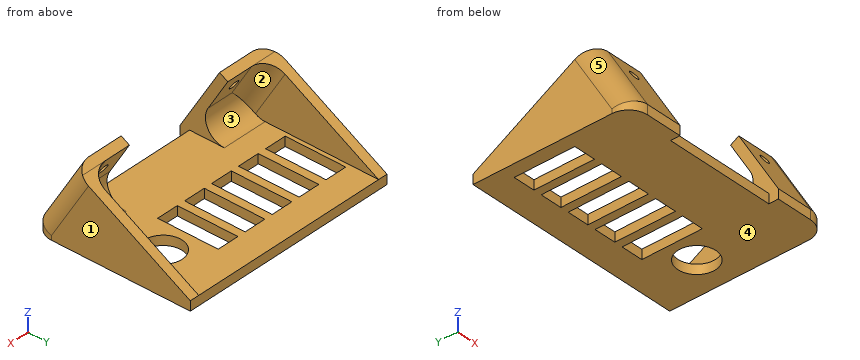
```python
from build123d import *

# Parameters (mm, degrees)
F3_W      = 7
F3_H      = 19.2
F3_R      = 6
F4_DEPTH  = 3
F7_DEPTH  = 3
F8_START  = -67
F8_DEPTH  = 3
F9_START  = -52.5
F9_DEPTH  = 17.5
F10_DEPTH = 17.5
F11_R     = 6
F13_R     = 1.5
F14_DEPTH = 5


with BuildPart() as f4:
    # F3 (on Top) → F4 (new body)
    with BuildSketch(Plane.XY):
        Polygon((35, 25), (-35, 25), (-35, -25), (-17.5, -25), (-17.5, -22), (17.5, -22), (17.5, -25), (35, -25), align=None)
        with Locations((-27.2, 6.1666666667)):
            Rectangle(F3_W, F3_H, mode=Mode.SUBTRACT)
        with Locations((-17.6, 6.1666666667)):
            Rectangle(F3_W, F3_H, mode=Mode.SUBTRACT)
        with Locations((-8, 6.1666666667)):
            Rectangle(F3_W, F3_H, mode=Mode.SUBTRACT)
        with Locations((1.6, 6.1666666667)):
            Rectangle(F3_W, F3_H, mode=Mode.SUBTRACT)
        with Locations((11.2, 6.1666666667)):
            Rectangle(F3_W, F3_H, mode=Mode.SUBTRACT)
        with Locations((23.5, 6.1666666667)):
            Circle(F3_R, mode=Mode.SUBTRACT)
    extrude(amount=F4_DEPTH)

    # F6 (on offset) → F7 (join)
    with BuildSketch(Plane.YZ.offset(35)):
        Polygon((-12.4875, 24.0638871947), (-25, 3), (-21.5106155706, 3), (-9.871334024, 22.5938871947), align=None)
        Polygon((-9.871334024, 22.5938871947), (-21.5106155706, 3), (25, 3), align=None)
    extrude(amount=-F7_DEPTH)

    # F6 (on offset) → F8 (join)
    with BuildSketch(Plane.YZ.offset(35).offset(F8_START)):
        Polygon((-12.4875, 24.0638871947), (-25, 3), (-21.5106155706, 3), (-9.871334024, 22.5938871947), align=None)
        Polygon((-9.871334024, 22.5938871947), (-21.5106155706, 3), (25, 3), align=None)
    extrude(amount=-F8_DEPTH)

    # F6 (on offset) → F9 (join)
    with BuildSketch(Plane.YZ.offset(35).offset(F9_START)):
        Polygon((-12.4875, 24.0638871947), (-25, 3), (-21.5106155706, 3), (-9.871334024, 22.5938871947), align=None)
    extrude(amount=-F9_DEPTH)

    # F6 (on offset) → F10 (join)
    with BuildSketch(Plane.YZ.offset(35)):
        Polygon((-12.4875, 24.0638871947), (-25, 3), (-21.5106155706, 3), (-9.871334024, 22.5938871947), align=None)
    extrude(amount=-F10_DEPTH)

    # F11
    f11_edges = [f4.edges().sort_by_distance(p)[0] for p in [
        (32, -15.690975, 12.796944),
        (-32, -15.690975, 12.796944),
        (-24.75, -21.510616, 3),
        (24.75, -21.510616, 3),
        (35, -18.74375, 13.531944),
        (-35, -18.74375, 13.531944),
        (-35, -25, 1.5),
        (35, -25, 1.5),
    ]]
    fillet(f11_edges, radius=F11_R)

    # F13 (on offset) → F14 (cut)
    with BuildSketch(Plane(origin=(0, -19.7965335432, 11.7596587786), x_dir=(1, 0, 0), z_dir=(0, -0.8597504977, 0.5107142857))):
        with Locations((-23.25, 8.1863943504)):
            Circle(F13_R)
        with Locations((23.25, 8.1863943504)):
            Circle(F13_R)
    extrude(amount=-F14_DEPTH, mode=Mode.SUBTRACT)


solid = f4.part
```
Could you check a few things on this model? Use its own coordinates, in mm. Face numbers are marked on the shaded views. A direction names the side the tool comes from. Round coordinates to 2 decimals unless told otherwise and drop trailing zeros. Loops run counter-clockwise (first coordinate to the right, second up) from the corner with the lowest first, then second, coordinate; pieces in that order, holes last. Notation, with made-up numbers: (-16, 15.25) -> (35, 15.25) arc R19 cw to (35, 35.25) -> close; hole circle Ø11 at (25, -30.75). An arc over 180 degrees is marked (long way). One line per question, with ' | ' between items.
(1) For the marked faces 1 and 2, which set-ups out of +Z, -Z, +X, -X, +Y, -Y let a thin tool reach every point of the face, with its end or its side?
Model answer:
face 1: +Z, -Z, +X, +Y, -Y | face 2: +Y
(2) If we section it at C-C on y = 13: List the corners of the cut face in (x, z) for me.
Model answer:
outline: (-35, 0) -> (-30.7, 0) -> (-30.7, 3) -> (-32, 3) -> (-32, 9.74) -> (-35, 9.74) -> close; (-23.7, 0) -> (-21.1, 0) -> (-21.1, 3) -> (-23.7, 3) -> close; (-14.1, 0) -> (-11.5, 0) -> (-11.5, 3) -> (-14.1, 3) -> close; (-4.5, 0) -> (-1.9, 0) -> (-1.9, 3) -> (-4.5, 3) -> close; (5.1, 0) -> (7.7, 0) -> (7.7, 3) -> (5.1, 3) -> close; (14.7, 0) -> (35, 0) -> (35, 9.74) -> (32, 9.74) -> (32, 3) -> (14.7, 3) -> close
(3) If we section it at A-A on x = -20: List the corners of the cut face in (y, z) for me, and give its area (3 significant figures).
Model answer:
outline: (-25, 0) -> (-3.43, 0) -> (-3.43, 3) -> (-10.97, 3) arc R6 cw to (-16.13, 12.06) -> (-9.87, 22.59) -> (-12.49, 24.06) -> (-25, 3) -> close; (15.77, 0) -> (25, 0) -> (25, 3) -> (15.77, 3) -> close | area: 189 mm^2
(4) For pin 1 Ø1 at (x, z) = (22.5, 16) entering from -Y; pin 2 Ø1.5 at (x, z) = (5.5, 2) entering from -Y; pin 3 Ø6 at (x, y) = (-26.5, 15) entering from +Z, each with a flat end and sliding along its axis, tell me the tip position at first contact or that it passes through.
Model answer:
pin 1: stops at y = -17.57 | pin 2: stops at y = -22 | pin 3: stops at z = 3
(5) If we section it at B-B on x = -9: List the corners of the cut face in (y, z) for me, and give its area (3 significant figures).
Model answer:
outline: (-22, 0) -> (-3.43, 0) -> (-3.43, 3) -> (-22, 3) -> close; (15.77, 0) -> (25, 0) -> (25, 3) -> (15.77, 3) -> close | area: 83.4 mm^2
(6) Thinking about a two-plate mould opening in X: for the marked faces 3, 4 and 5, which applies, released by +X, released by -X, zero draft, split by the parting line, or undercut?
Model answer:
face 3: undercut | face 4: zero draft | face 5: released by -X
(7) If we section it at D-D on x = 23.5: List the corners of the cut face in (y, z) for me, and give its area (3 significant figures).
Model answer:
outline: (-25, 0) -> (0.17, 0) -> (0.17, 3) -> (-10.97, 3) arc R6 cw to (-16.13, 12.06) -> (-13.79, 15.99) -> (-16.37, 17.53) -> (-25, 3) -> close; (-14.86, 20.07) -> (-12.28, 18.54) -> (-9.87, 22.59) -> (-12.49, 24.06) -> close; (12.17, 0) -> (25, 0) -> (25, 3) -> (12.17, 3) -> close | area: 201 mm^2
(8) If I drill on probe 1 along Y at (x, z) = (23.5, 1.8); probe 2 along X at (y, z) = (-4.5, 4.5); probe 3 along X at (y, z) = (-16.5, 3.75), over which ranges is the centre line in solid material (lowest first)?
Model answer:
probe 1: y = -25 to 0.17, 12.17 to 25 | probe 2: x = -35 to -32, 32 to 35 | probe 3: x = -35 to -17.5, 17.5 to 35
